Verification items for this drawing (mm, ordinates from the low corner). Round coordinates to 2 decimals unless told otherwise and drop trailing zeros. Loops run counter-clockwise (first coordinate to the right, second up) from the corner with the lowest first, then second, coordinate; pieces in that order, holes last. Notation, with made-up numbers: (-22.5, 17.25) - (6.5, 17.25) arc R11 ccw to (6.5, 30.25) - close; hole circle Ø3 at (-6.5, 70.25). An arc over 180 degrees is marked (long way). Answer in a Markdown table with one row per item. Add a question column.
(1) Cross-section at C-C on x = 83. Enter the section's corners in (y, z).
(2) Cross-section at B-B on x = 172.5. Enter the section's corners in (y, z), then the cut area to 3 significant figures.
(3) Cross-section at D-D on z = 410. Enter the section's corners in (x, y).
(4) Gauge pin test, flat ends, axial feed: pin 1 (4.5 mm diameter, centred on y = 687.5, z = 500, fed in from -X); pin 2 (8 mm diameter, centred on x = 187.5, z = 287.5, fed in from +Y); pin 3 (16.5 mm diameter, centred on x = 141, y = 4.5, fed in from +Z). Record the tip position at first contact, or that the pin passes through.
(5) Thickness scan on line 1 along Y through (x, z) = (82.5, 170.5). Record the ranges inside material, lowest first.
(6) Cross-section at A-A on z = 120. Enter the section's corners in (x, y).
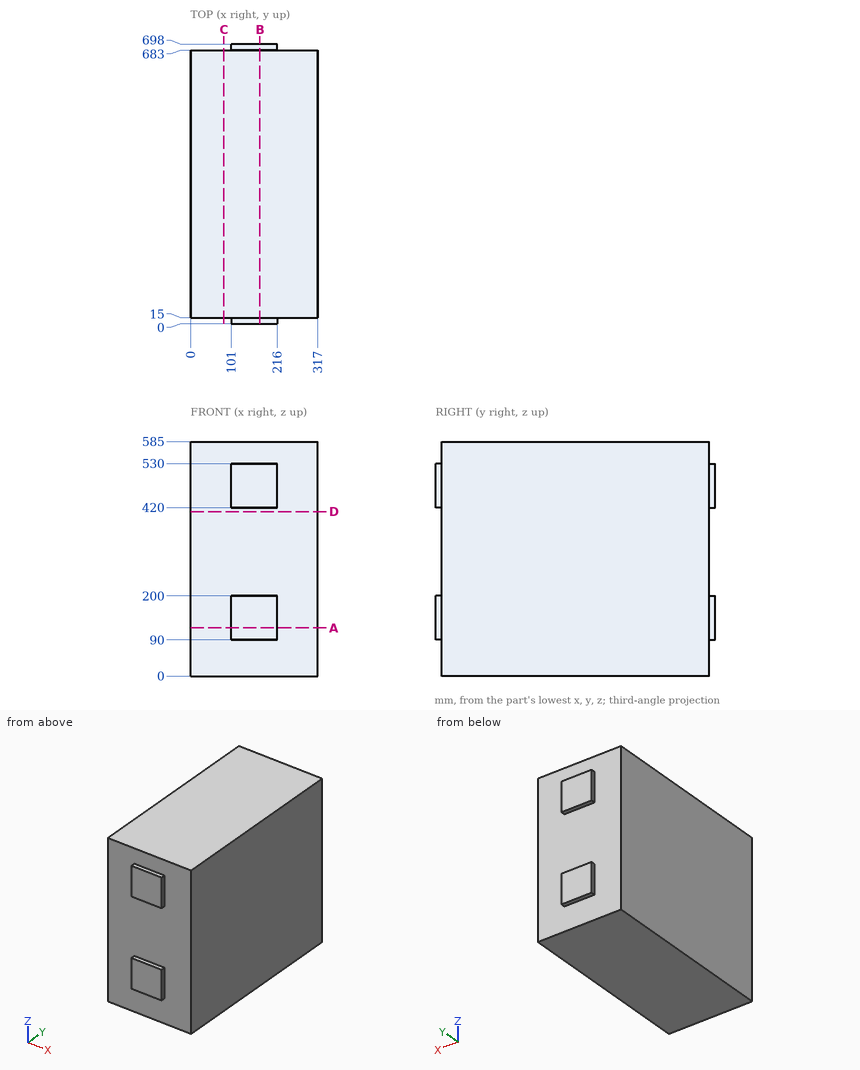
Answers:
| question | item | result |
|---|---|---|
| 1 | outline | (15, 0) - (683, 0) - (683, 585) - (15, 585) - close |
| 2 | outline | (0, 90) - (15, 90) - (15, 0) - (683, 0) - (683, 90) - (698, 90) - (698, 200) - (683, 200) - (683, 420) - (698, 420) - (698, 530) - (683, 530) - (683, 585) - (15, 585) - (15, 530) - (0, 530) - (0, 420) - (15, 420) - (15, 200) - (0, 200) - close |
| 2 | area | 397,000 mm^2 |
| 3 | outline | (0, 15) - (317, 15) - (317, 683) - (0, 683) - close |
| 4 | pin 1 | stops at x = 101 |
| 4 | pin 2 | stops at y = 683 |
| 4 | pin 3 | stops at z = 530 |
| 5 | line 1 | y = 15 to 683 |
| 6 | outline | (0, 15) - (101, 15) - (101, 0) - (216, 0) - (216, 15) - (317, 15) - (317, 683) - (216, 683) - (216, 698) - (101, 698) - (101, 683) - (0, 683) - close |
